Autodesk Inventor part; units mm, degrees
ref_plane "YZ Plane" through (0, 0, 0) normal (1, 0, 0) x (0, 1, 0)
ref_plane "XZ Plane" through (0, 0, 0) normal (0, 1, 0) x (-1, 0, 0)
ref_plane "XY Plane" through (0, 0, 0) normal (0, 0, 1) x (1, 0, 0)
sketch "MASTER SKETCH" plane through (0, 0, 0) normal (0, 0, 1) x (1, 0, 0)
  circle A0 centre (0, 0) radius 22.86
  circle A1 centre (-31.6504, 3.081) radius 8.89
  circle A2 centre (-31.6504, 3.081) radius 20.32
  circle A3 centre (-60.6627, 6.8802) radius 8.89
  circle A4 centre (-58.2971, 5.0584) radius 6.35
  circle A5 centre (-60.6627, 6.8802) radius 25.4
  circle A6 centre (-58.2971, 5.0584) radius 25.4 construction
  line L0 (-44.0087, 26.0584) -> (-77.3167, -12.298) construction
  line L1 (-68.9445, 30.8921) -> (-52.3809, -17.1317) construction
  line L2 (-85.8186, 10.3933) -> (-36.0162, 0.7394) construction
  circle A7 centre (-44.0087, 26.0584) radius 2
  arc A8 (-68.9445, 30.8921) -> (-69.3394, 27.9326) centre (-44.0087, 26.0584) ccw construction
  arc A9 (-70.9079, 31.2727) -> (-71.334, 28.0802) centre (-44.0087, 26.0584) ccw
  arc A10 (-66.981, 30.5115) -> (-67.3449, 27.785) centre (-44.0087, 26.0584) ccw
  arc A11 (-66.981, 30.5115) -> (-70.9079, 31.2727) centre (-68.9445, 30.8921) ccw
  arc A12 (-71.334, 28.0802) -> (-67.3449, 27.785) centre (-69.3394, 27.9326) ccw
  arc A13 (-85.8186, 10.3933) -> (-83.6914, 5.5953) centre (-44.0087, 26.0584) ccw construction
  arc A14 (-87.6914, 9.6916) -> (-85.469, 4.6787) centre (-44.0087, 26.0584) ccw
  arc A15 (-83.9457, 11.0951) -> (-81.9139, 6.5119) centre (-44.0087, 26.0584) ccw
  arc A16 (-83.9457, 11.0951) -> (-87.6914, 9.6916) centre (-85.8186, 10.3933) ccw
  arc A17 (-85.469, 4.6787) -> (-81.9139, 6.5119) centre (-83.6914, 5.5953) ccw
  arc A18 (-77.3167, -12.298) -> (-72.5856, -15.9416) centre (-44.0087, 26.0584) ccw construction
  arc A19 (-78.6281, -13.8081) -> (-73.7107, -17.5951) centre (-44.0087, 26.0584) ccw
  arc A20 (-76.0054, -10.7879) -> (-71.4605, -14.288) centre (-44.0087, 26.0584) ccw
  arc A21 (-76.0054, -10.7879) -> (-78.6281, -13.8081) centre (-77.3167, -12.298) ccw
  arc A22 (-73.7107, -17.5951) -> (-71.4605, -14.288) centre (-72.5856, -15.9416) ccw
  arc A23 (-52.3809, -17.1317) -> (-47.2548, -17.8157) centre (-44.0087, 26.0584) ccw construction
  arc A24 (-52.7615, -19.0951) -> (-47.4024, -19.8103) centre (-44.0087, 26.0584) ccw
  arc A25 (-52.0003, -15.1682) -> (-47.1072, -15.8212) centre (-44.0087, 26.0584) ccw
  arc A26 (-52.0003, -15.1682) -> (-52.7615, -19.0951) centre (-52.3809, -17.1317) ccw
  arc A27 (-47.4024, -19.8103) -> (-47.1072, -15.8212) centre (-47.2548, -17.8157) ccw
  arc A28 (-36.0162, 0.7394) -> (-33.1003, 1.8522) centre (-44.0087, 26.0584) ccw construction
  arc A29 (-35.4141, -1.1679) -> (-32.2786, 0.0288) centre (-44.0087, 26.0584) ccw
  arc A30 (-36.6183, 2.6466) -> (-33.922, 3.6756) centre (-44.0087, 26.0584) ccw
  arc A31 (-36.6183, 2.6466) -> (-35.4141, -1.1679) centre (-36.0162, 0.7394) ccw
  arc A32 (-32.2786, 0.0288) -> (-33.922, 3.6756) centre (-33.1003, 1.8522) ccw
  line L3 (-91.0627, 30.0584) -> (30.5868, 30.0584)
  line L4 (30.5868, 30.0584) -> (30.5868, -19.9416)
  line L5 (30.5868, -19.9416) -> (-91.0627, -19.9416)
  line L6 (-91.0627, -19.9416) -> (-91.0627, 30.0584)
  circle A33 centre (0, 0) radius 14.2875 construction
  circle A34 centre (25.5868, -14.9416) radius 3
  circle A35 centre (25.5868, 25.0584) radius 3
  circle A36 centre (-51.8755, -14.9416) radius 3
  line L7 (-91.0627, 25.3566) -> (30.5868, 25.3566) construction
  circle A37 centre (-15.8118, 25.0584) radius 3
  line L8 (-58.2971, 5.0584) -> (-60.6627, 6.8802) construction
  line L9 (-52.0979, 13.108) -> (-54.4635, 14.9298)
  line L10 (-66.8619, -1.1693) -> (-64.4963, -2.9911)
  arc A38 (-64.4963, -2.9911) -> (-52.0979, 13.108) centre (-58.2971, 5.0584) ccw
  arc A39 (-54.4635, 14.9298) -> (-66.8619, -1.1693) centre (-60.6627, 6.8802) ccw
  circle A40 centre (0, 0) radius 24.13 construction
  circle A41 centre (-31.6504, 3.081) radius 21.59 construction
  line L11 (-67.7771, -2.3578) -> (-65.4116, -4.1796)
  arc A42 (-65.4116, -4.1796) -> (-51.1827, 14.2964) centre (-58.2971, 5.0584) ccw
  line L12 (-51.1827, 14.2964) -> (-53.5482, 16.1182)
  arc A43 (-53.5482, 16.1182) -> (-67.7771, -2.3578) centre (-60.6627, 6.8802) ccw
  point P0 (-60.0285, -7.7006)
  point P1 (-59.4799, 5.9693)
  dimension "d0" = 45.72
  dimension "d1" = 17.78
  dimension "d2" = 40.64
  dimension "d4" = 17.78
  dimension "d5" = 12.7
  dimension "d6" = 50.8
  dimension "d9" = 50.8
  dimension "d10" = 60
  dimension "d11" = 60
  dimension "d12" = 4
  dimension "d13" = 4
  dimension "d14" = 4
  dimension "d15" = 4
  dimension "d16" = 4
  dimension "d17" = 4
  dimension "d19" = 28.575
  dimension "d28" = 6
  dimension "d29" = 6
  dimension "d30" = 6
  dimension "d39" = 31.8
  dimension "d42" = 29.26
  dimension "d43" = 26.72
  dimension "d70" = 2
  dimension "d73" = 6
  dimension "d84" = 2
  dimension "d85" = 5
  dimension "d89" = 20.32
  dimension "d108" = 1.27
  dimension "d109" = 1.27
  dimension "d110" = 2.5
  dimension "d111" = 2.5
  dimension "d113" = 2.5
  dimension "d114" = 2
  dimension "d129" = 1.5
  dimension "d133" = 2.5
  dimension "d136" = 50
  dimension "d139" = 2
  dimension "d140" = 2.5
  dimension "d141" = 2
  dimension "d142" = 2
sketch "Sketch2" plane through (0, 0, 0) normal (0, 0, 1) x (1, 0, 0)
  line L0 (-91.0627, 30.0584) -> (30.5868, 30.0584)
  line L1 (-91.0627, -19.9416) -> (-91.0627, 30.0584)
  line L2 (30.5868, 30.0584) -> (30.5868, -19.9416)
  line L3 (30.5868, -19.9416) -> (-91.0627, -19.9416)
  line L4 (-91.0627, 30.0584) -> (30.5868, 30.0584)
  line L5 (30.5868, 30.0584) -> (30.5868, -19.9416)
  line L6 (30.5868, -19.9416) -> (-91.0627, -19.9416)
  line L7 (-91.0627, -19.9416) -> (-91.0627, 30.0584)
  point P0 (0, 0)
extrude "Extrusion1" [suppressed]
sketch "Sketch3" plane through (0, 0, 0) normal (0, 0, -1) x (-1, 0, 0)
  arc A0 (47.1072, -15.8212) -> (47.4024, -19.8103) centre (47.2548, -17.8157) ccw
  arc A1 (47.1072, -15.8212) -> (52.0003, -15.1682) centre (44.0087, 26.0584) ccw
  arc A2 (47.4024, -19.8103) -> (52.7615, -19.0951) centre (44.0087, 26.0584) ccw
  arc A3 (52.7615, -19.0951) -> (52.0003, -15.1682) centre (52.3809, -17.1317) ccw
  line L0 (91.0627, 30.0584) -> (91.0627, -19.9416)
  line L1 (-30.5868, 30.0584) -> (91.0627, 30.0584)
  line L2 (-30.5868, -19.9416) -> (-30.5868, 30.0584)
  line L3 (91.0627, -19.9416) -> (-30.5868, -19.9416)
  arc A4 (71.4605, -14.288) -> (73.7107, -17.5951) centre (72.5856, -15.9416) ccw
  arc A5 (73.7107, -17.5951) -> (78.6281, -13.8081) centre (44.0087, 26.0584) ccw
  arc A6 (71.4605, -14.288) -> (76.0054, -10.7879) centre (44.0087, 26.0584) ccw
  arc A7 (78.6281, -13.8081) -> (76.0054, -10.7879) centre (77.3167, -12.298) ccw
  arc A8 (81.9139, 6.5119) -> (83.9457, 11.0951) centre (44.0087, 26.0584) ccw
  arc A9 (81.9139, 6.5119) -> (85.469, 4.6787) centre (83.6914, 5.5953) ccw
  arc A10 (85.469, 4.6787) -> (87.6914, 9.6916) centre (44.0087, 26.0584) ccw
  arc A11 (87.6914, 9.6916) -> (83.9457, 11.0951) centre (85.8186, 10.3933) ccw
  arc A12 (71.334, 28.0802) -> (70.9079, 31.2727) centre (44.0087, 26.0584) ccw
  arc A13 (67.3449, 27.785) -> (66.981, 30.5115) centre (44.0087, 26.0584) ccw
  arc A14 (70.9079, 31.2727) -> (66.981, 30.5115) centre (68.9445, 30.8921) ccw
  arc A15 (67.3449, 27.785) -> (71.334, 28.0802) centre (69.3394, 27.9326) ccw
  arc A16 (66.8619, -1.1693) -> (54.4635, 14.9298) centre (60.6627, 6.8802) ccw
  arc A17 (52.0979, 13.108) -> (64.4963, -2.9911) centre (58.2971, 5.0584) ccw
  line L4 (52.0979, 13.108) -> (54.4635, 14.9298)
  line L5 (66.8619, -1.1693) -> (64.4963, -2.9911)
  point P0 (0, 0)
extrude "Extrusion2" [suppressed]
sketch "Sketch4" plane through (0, 0, 0) normal (0, 0, -1) x (-1, 0, 0)
  circle A0 centre (-25.5868, 25.0584) radius 3
  circle A1 centre (15.8118, 25.0584) radius 3
  circle A2 centre (51.8755, -14.9416) radius 3
  circle A3 centre (-25.5868, -14.9416) radius 3
  point P0 (0, 0)
sketch "Sketch5" plane through (0, 0, 0) normal (0, 0, -1) x (-1, 0, 0)
  circle A0 centre (0, 0) radius 22.86
hole "Hole1" [suppressed]
hole "Hole2" [suppressed]
sketch "Sketch6" plane through (0, 0, 0) normal (0, 0, -1) x (-1, 0, 0)
  line L0 (91.0627, 25.3566) -> (-30.5868, 25.3566) construction
  circle A0 centre (44.0087, 26.0584) radius 2
  point P0 (0, 0)
hole "Hole3" [suppressed]
sketch "Sketch7" plane through (0, 0, 0) normal (0, 0, -1) x (-1, 0, 0)
  circle A0 centre (31.6504, 3.081) radius 20.32
  point P0 (0, 0)
hole "Hole4" [suppressed]
sketch "Sketch8" plane through (0, 0, 0) normal (0, 0, -1) x (-1, 0, 0)
  arc A0 (52.0979, 13.108) -> (64.4963, -2.9911) centre (58.2971, 5.0584) ccw
  line L0 (66.8619, -1.1693) -> (64.4963, -2.9911)
  arc A1 (66.8619, -1.1693) -> (54.4635, 14.9298) centre (60.6627, 6.8802) ccw
  line L1 (52.0979, 13.108) -> (54.4635, 14.9298)
  arc A2 (67.7771, -2.3578) -> (53.5482, 16.1182) centre (60.6627, 6.8802) ccw
  line L2 (51.1827, 14.2964) -> (53.5482, 16.1182)
  line L3 (67.7771, -2.3578) -> (65.4116, -4.1796)
  arc A3 (51.1827, 14.2964) -> (65.4116, -4.1796) centre (58.2971, 5.0584) ccw
  point P0 (0, 0)
extrude "Extrusion3" [suppressed]
sketch "Sketch11" plane through (0, 0, 0) normal (0, 0, 1) x (1, 0, 0)
  line L0 (30.5868, -19.9416) -> (30.5868, 30.0584)
  line L1 (30.5868, 30.0584) -> (30.5868, -19.9416)
  line L2 (30.5868, -19.9416) -> (-61.3292, -19.9416)
  line L3 (-91.0627, -19.9416) -> (30.5868, -19.9416)
  line L4 (-61.3292, -19.9416) -> (-32.4617, 30.0584)
  line L5 (30.5868, 30.0584) -> (-91.0627, 30.0584)
  line L6 (-32.4617, 30.0584) -> (30.5868, 30.0584)
  circle A0 centre (-44.0087, 26.0584) radius 2
  point P0 (0, 0)
  dimension "d147" = 120
  dimension "d148" = 8
extrude "Extrusion5" add sketch "Sketch11" against normal blind 5 contours L2 L4 L5 L0
sketch "Sketch12" plane through (0, 0, 0) normal (0, 0, 1) x (1, 0, 0)
  circle A0 centre (-15.8118, 25.0584) radius 3
  circle A1 centre (25.5868, 25.0584) radius 3
  circle A2 centre (25.5868, -14.9416) radius 3
  circle A3 centre (-51.8755, -14.9416) radius 3
  point P0 (0, 0)
hole "Hole5" at (-15.8118, 25.0584, 0) at (-51.8755, -14.9416, 0) at (25.5868, -14.9416, 0) at (25.5868, 25.0584, 0) direction (0, 0, -1) diameter 4.5 end through all counterbore diameter 6 counterbore depth 1
sketch "Sketch13" plane through (0, 0, 0) normal (0, 0, 1) x (1, 0, 0)
  circle A0 centre (0, 0) radius 14.2875 construction
hole "Hole6" at (0, 0, 0) direction (0, 0, -1) diameter 28.575 end through all
sketch "Sketch14" plane through (0, 0, 0) normal (0, 0, 1) x (1, 0, 0)
  circle A0 centre (-31.6504, 3.081) radius 8.89
  point P0 (0, 0)
hole "Hole7" at (-31.6504, 3.081, 0) direction (0, 0, -1) diameter 8 depth 5 counterbore diameter 22 counterbore depth 3
sketch "Sketch15" plane through (0, 0, -5) normal (0, 0, -1) x (-1, 0, 0)
  circle A0 centre (-25.5868, 25.0584) radius 2.25
  circle A1 centre (-25.5868, -14.9416) radius 2.25
  circle A2 centre (51.8755, -14.9416) radius 2.25
  circle A3 centre (15.8118, 25.0584) radius 2.25
  point P0 (0, 0)
hole "Hole8" at (25.5868, 25.0584, -5) at (-15.8118, 25.0584, -5) at (25.5868, -14.9416, -5) at (-51.8755, -14.9416, -5) direction (0, 0, 1) diameter 4 end through all countersink diameter 8 countersink angle 90
sketch "Sketch16" plane through (0, 0, -5) normal (0, 0, -1) x (-1, 0, 0)
  circle A0 centre (-25.5868, 25.0584) radius 4 construction
  circle A1 centre (-25.5868, -14.9416) radius 4 construction
  circle A2 centre (15.8118, 25.0584) radius 4 construction
  circle A3 centre (51.8755, -14.9416) radius 4 construction
  circle A4 centre (31.6504, 3.081) radius 4
  point P0 (0, 0)
  point P1 (-25.5868, -2.9416)
  point P2 (-25.5868, 13.0584)
  point P3 (15.8118, -14.9416)
  point P4 (0, 22.5584)
  point P5 (-15.5868, -14.9416)
  point P6 (31.6504, -14.9416)
  point P7 (31.6504, 22.5584)
  dimension "d181" = 10
  dimension "d182" = 12
  dimension "d183" = 12
  dimension "d191" = 2.5
hole "Hole9" at (25.5868, -2.9416, -5) at (25.5868, 13.0584, -5) at (-15.8118, -14.9416, -5) at (0, 22.5584, -5) at (15.5868, -14.9416, -5) at (-31.6504, -14.9416, -5) at (-31.6504, 22.5584, -5) direction (0, 0, 1) diameter 3.242 depth 10
equation "\"d0\" = SR2PD"
equation "\"d1\" = SR1PD"
equation "\"d2\" = FirstReductionPD"
equation "\"d4\" = Pinion4inPD"
equation "\"d5\" = PinionPD"
equation "\"PinionPD\" = 12.7"
equation "\"FirstReductionPD\" = 40.64"
equation "\"HighGearPD\" = 20.32"
equation "\"LowGearPD\" = 17.78"
equation "\"HighGearDogPD\" = 63.5"
equation "\"LowGearDogPD\" = 76.2"
equation "\"SR1PD\" = 17.78"
equation "\"SR2PD\" = 45.72"
equation "\"Pinion4inPD\" = 17.78"
properties part number "GEARBOX FRONT PLATE" material "Aluminum 6061"
CAD build for the part. Positions are in the model's coordinates, mm. A direction names the side the tool comes from. Give positions to 0.01 mm unless a question says otherwise; leave off trailing zeros. Order: outer loops, then holes, each group sorted by start corner. A loop starts at its lowest first (then second) coordinate and runs counter-clockwise, first axis right, second up.
(1) Saw through at B-B, the plane y = 9. Give the cut face in (x, z).
(2) Flat gauge pins, fed straight in: pin 1 (1.5 mm diameter, centred on y = 25, z = -3.5, fed in from -X); pin 2 (5.5 mm diameter, centred on x = -51.88, y = -14.94, fed in from +Z); pin 3 (1.9 mm diameter, centred on x = -31.65, y = -14.94, fed in from +Z). Where does each tip first touch, or does it go through?
(3) Tool access for faces 3 (the cylindrical face through (26.74, 22.29, -0.51)), 4 (the conical face through (27.926, -15.249, -3.359)): list every direction of +Z, -Z, +X, -X, +Y, -Y with a clear straight run to the whole face (end or side of a thin tool).
(4) Saw through at A-A, the plane x = 0. Give the cut face in (y, z), then the cut area to 3 significant figures.
(5) Saw through at D-D, the plane x = -24. Give the cut face in (y, z), then the cut area to 3 significant figures.
(6) Mould opens along X. For faces 1 (the flat face through (23, 25, -1)), 2 (the flat face through (0, 30.058, -2)) say: released by +X, released by -X, zero draft, split by the parting line, or undercut.
(7) Saw through at C-C, the plane y = 0. Give the cut face in (x, z), then the cut area to 3 significant figures.
(8) Drill centre lines: L1, parallel to X at y = 23.5, z = -1.85; L2, parallel to Y at x = 0, z = -1.85; L3, parallel to X at y = -17, z = -4.4. Where is each one in solid material? Low to high.
Results found:
1. outline: (-44.62, -5) - (-11.1, -5) - (-11.1, 0) - (-22.38, 0) - (-22.38, -3) - (-40.92, -3) - (-40.92, 0) - (-44.62, 0) - close; (11.1, -5) - (30.59, -5) - (30.59, 0) - (11.1, 0) - close
2. pin 1: stops at x = -35.82
2. pin 2: stops at z = -1
2. pin 3: passes through
3. face 3: +Z
3. face 4: -Z
4. outline: (-19.94, -5) - (-14.29, -5) - (-14.29, 0) - (-19.94, 0) - close; (14.29, -5) - (20.94, -5) - (20.94, 0) - (14.29, 0) - close; (24.18, -5) - (30.06, -5) - (30.06, 0) - (24.18, 0) - close
4. area: 90.9 mm2
5. outline: (-19.94, -5) - (30.06, -5) - (30.06, 0) - (10.98, 0) - (10.98, -3) - (-4.82, -3) - (-4.82, 0) - (-19.94, 0) - close
5. area: 203 mm2
6. face 1: undercut
6. face 2: zero draft
7. outline: (-49.82, -5) - (-34.2, -5) - (-34.2, -3) - (-42.21, -3) - (-42.21, 0) - (-49.82, 0) - close; (-29.1, -5) - (-14.29, -5) - (-14.29, 0) - (-21.09, 0) - (-21.09, -3) - (-29.1, -3) - close; (14.29, -5) - (30.59, -5) - (30.59, 0) - (14.29, 0) - close
7. area: 186 mm2
8. L1: x = -36.25 to -32.97, -30.33 to -17.43, -14.19 to -1.32, 1.32 to 23.96, 27.21 to 30.59
8. L2: y = -19.94 to -14.29, 14.29 to 20.94, 24.18 to 30.06
8. L3: x = -59.63 to -54.58, -49.17 to 22.88, 28.29 to 30.59
